Geometry check sheet. Reference: the model listing, model coordinates, mm. Face numbers are marked on the shaded views. A direction names the side the tool comes from. Give positions to 0.01 mm unless a question says otherwise; leave off trailing zeros. Write each loop counter-clockwise with the first axis right and the second up, starting at its lowest first coordinate (ties: lowest second). Pieces come first, ordered by that corner, then holes. Notation, with made-up numbers: (27, 8) -> (42, 8) arc R12 cw to (42, 31) -> close; hole circle Ø2 at (-39.75, 28.25). An arc over 180 degrees is marked (long way). Write item = value, one per line. Start each with the question number.
1. Mould release check, pull along X, two halves, no side actions. Record for the marked faces 1, 2, 3 and 4: pulls with the +X half, pulls with the -X half, needs draft (parallel to the pull), parting line crosses it, or undercut.
2. Depth check by flat-ended pin: P1, Ø3.5, axis at x = -2.5, z = 4, coming from the +Y side; P2, Ø0.9, axis at x = -3.5, z = 5, coming from the -Y side (3 decimals); P3, Ø1.3, axis at x = -4.5, y = 0, coming from the +Z side; P4, Ø2, axis at x = -5.5, z = 5, coming from the -Y side (3 decimals). Enter the tip coordinate at first touch or a pass-through.
3. Set-up check for the marked faces 5, 6, 7, 8 and 9: record each of +Z, -Z, +X, -X, +Y, -Y from which the full face is reachable in a straight line by a thin tool's end or side.
4. Cross-section at C-C, the plane z = -0.75. Record the cut outline in (x, y), plus the area to 3 significant figures.
5. Cross-section at A-A, the plane y = 0. Record the cut outline in (x, z).
6. Thickness scan on line 1 along Y through (x, z) = (9.75, 9.15); line 2 along Z through (x, y) = (6, 4.25); line 3 along Y through (x, z) = (-4.75, 1.75) (3 decimals). Record the ranges inside material, lowest first.
7. Cross-section at D-D, the plane x = 9.5. Record the cut outline in (y, z), plus the area to 3 significant figures.
8. Cross-section at B-B, the plane x = 3.25. Record the cut outline in (y, z).
```python
from build123d import *

# Parameters (mm, degrees)
BOSS_EXTRUDE1_DEPTH  = 8
SKETCH2_R            = 2.5
BOSS_EXTRUDE3_DEPTH  = 2.5
CUT_EXTRUDE2_DEPTH   = 19.656433207
FILLET5_R            = 1
FILLET6_R            = 2.5
FILLET5_OF_MIRROR2_R = 1
FILLET6_OF_MIRROR2_R = 2.5


with BuildPart() as part:
    # Sketch1 → Boss-Extrude1 (new body)
    with BuildSketch(Plane.XY):
        Polygon((1.25, -4.5), (-1.25, -4.5), (-1.25, -1.475), (-4.3, -1.475), (-4.3, -2.225), (-6.25, -2.225), (-6.25, 2.225), (-4.3, 2.225), (-4.3, 1.475), (-1.25, 1.475), (-1.25, 4.5), (1.25, 4.5), align=None)
    extrude(amount=BOSS_EXTRUDE1_DEPTH)

    # Sketch2 → Boss-Extrude3 (add)
    with BuildSketch(Plane.XY):
        with BuildLine():
            Line((9.75, -4.5), (-1.25, -4.5))
            Line((-1.25, -4.5), (-1.25, 4.5))
            Line((-1.25, 4.5), (9.75, 4.5))
            ThreePointArc((9.75, 4.5), (14.25, 0), (9.75, -4.5))
        make_face()
        with Locations((9.75, 0)):
            Circle(SKETCH2_R, mode=Mode.SUBTRACT)
    boss_extrude3 = extrude(amount=-BOSS_EXTRUDE3_DEPTH)

    # Sketch5 → Cut-Extrude2 (cut, symmetric)
    with BuildSketch(Plane(origin=(0, 4.5, 0), x_dir=(1, 0, 0), z_dir=(0, 1, 0))):
        Polygon((-1.25, 2.5), (1.25, 2.5), (-1.25, 0), align=None)
    cut_extrude2 = extrude(amount=CUT_EXTRUDE2_DEPTH, both=True, mode=Mode.SUBTRACT)

    # Fillet5
    fillet5_edges = [part.edges().sort_by_distance(p)[0] for p in [
        (1.25, 0, 0),
    ]]
    fillet(fillet5_edges, radius=FILLET5_R)

    # Fillet6
    fillet6_edges = [part.edges().sort_by_distance(p)[0] for p in [
        (1.25, 0, -2.5),
    ]]
    fillet(fillet6_edges, radius=FILLET6_R)

    # Mirror2: Boss-Extrude3, Cut-Extrude2 across plane
    add(boss_extrude3.mirror(Plane(origin=(0, 0, 4), x_dir=(1, 0, 0), z_dir=(0, 0, -1))))
    add(cut_extrude2.mirror(Plane(origin=(0, 0, 4), x_dir=(1, 0, 0), z_dir=(0, 0, -1))), mode=Mode.SUBTRACT)

    # Fillet5 of Mirror2
    fillet5_of_mirror2_edges = [part.edges().sort_by_distance(p)[0] for p in [
        (1.25, 0, 8),
    ]]
    fillet(fillet5_of_mirror2_edges, radius=FILLET5_OF_MIRROR2_R)

    # Fillet6 of Mirror2
    fillet6_of_mirror2_edges = [part.edges().sort_by_distance(p)[0] for p in [
        (1.25, 0, 10.5),
    ]]
    fillet(fillet6_of_mirror2_edges, radius=FILLET6_OF_MIRROR2_R)


solid = part.part
```
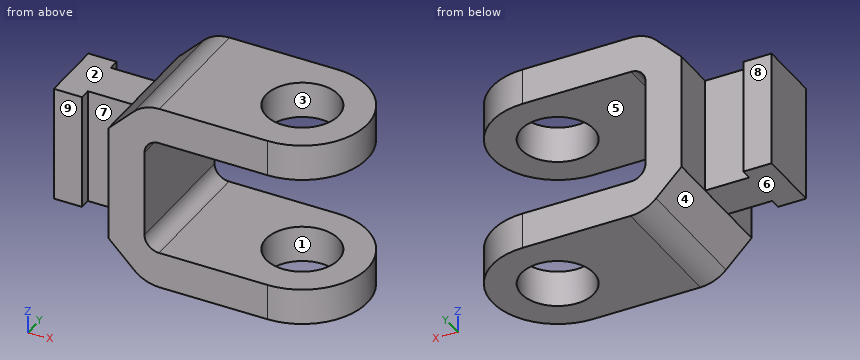
Answers:
q1.face_1 = undercut
q1.face_2 = needs draft
q1.face_3 = undercut
q1.face_4 = pulls with the -X half
q2.P1 = 4.5
q2.P2 = -1.475
q2.P3 = 8
q2.P4 = -2.225
q3.face_5 = +X, +Y, -Y
q3.face_6 = -Z, -X, +Y, -Y
q3.face_7 = +Z, -Z, -Y
q3.face_8 = +Z, -Z, -X, +Y
q3.face_9 = +Z, -Z, -X, -Y
q4.outline = (-0.5, -4.5) -> (9.75, -4.5) arc R4.5 ccw to (9.75, 4.5) -> (-0.5, 4.5) -> close; hole circle Ø5 at (9.75, 0)
q4.area = 104 mm^2
q5.outline = (-6.25, 0) -> (-1.25, 0) -> (0.52, -1.77) arc R2.5 ccw to (2.29, -2.5) -> (7.25, -2.5) -> (7.25, 0) -> (2.25, 0) arc R1 cw to (1.25, 1) -> (1.25, 7) arc R1 cw to (2.25, 8) -> (7.25, 8) -> (7.25, 10.5) -> (2.29, 10.5) arc R2.5 ccw to (0.52, 9.77) -> (-1.25, 8) -> (-6.25, 8) -> close; (12.25, -2.5) -> (14.25, -2.5) -> (14.25, 0) -> (12.25, 0) -> close; (12.25, 8) -> (14.25, 8) -> (14.25, 10.5) -> (12.25, 10.5) -> close
q6.line_1 = -4.5 to -2.5, 2.5 to 4.5
q6.line_2 = -2.5 to 0, 8 to 10.5
q6.line_3 = -2.225 to 2.225
q7.outline = (-4.5, -2.5) -> (-2.49, -2.5) -> (-2.49, 0) -> (-4.5, 0) -> close; (-4.5, 8) -> (-2.49, 8) -> (-2.49, 10.5) -> (-4.5, 10.5) -> close; (2.49, -2.5) -> (4.5, -2.5) -> (4.5, 0) -> (2.49, 0) -> close; (2.49, 8) -> (4.5, 8) -> (4.5, 10.5) -> (2.49, 10.5) -> close
q7.area = 20.1 mm^2
q8.outline = (-4.5, -2.5) -> (4.5, -2.5) -> (4.5, 0) -> (-4.5, 0) -> close; (-4.5, 8) -> (4.5, 8) -> (4.5, 10.5) -> (-4.5, 10.5) -> close
